Input: part model. Units: mm. Frame: model coordinates. Face numbers are marked on the shaded views. A direction names the side the tool comes from. Give positions to 0.01 mm unless a question says otherwise; leave off trailing zeros. Write each loop counter-clockwise with the first axis right and the second up, starting at its lowest first coordinate (ties: lowest second). Pieces come first, ordered by that corner, then holes. Notation, with made-up numbers: (45.25, 33.25) - (55.25, 33.25) arc R14 cw to (55.25, 46.25) - close; hole circle Ø8 at (60.5, -10.5). An arc over 180 degrees is marked (long way). Use a Markdown table: item, result. Add a question column.
1. Section query A-A, the plane x = -40. Return loops of the section in (y, z) (3 decimals), plus the area to 3 significant figures.
2. Pin query (flat end, axial travel): pin 1 (1.8 mm diameter, centred on y = 25, z = -2.5, fed in from +X); pin 2 (7.5 mm diameter, centred on x = 20.5, y = -31, fed in from +Z); pin 3 (3 mm diameter, centred on x = 42, z = -3.5, fed in from +Y). Return the tip coordinate at first contact, or that it passes through.
3. Set-up query: the marked faces 1, 2 and 3. Return all of +Z, -Z, +X, -X, +Y, -Y with unobstructed straight access to the full face (end or side cutting, diameter ignored); none if empty.
4. Material intervals for probe 1 along Y at (x, z) = (21.2, -4.7); probe 2 along Y at (x, z) = (-21.2, -3.95); probe 3 along Z at (x, y) = (30, 24.5), sorted ascending.
5. Section query B-B, the plane y = 0. Return loops of the section in (x, z) (3 decimals).
6. Section query C-C, the plane x = 21.2. Return loops of the section in (y, z).
7. Section query D-D, the plane x = -21.2. Return loops of the section in (y, z), plus the area to 3 significant figures.
```python
from build123d import *

# Parameters (mm, degrees)
F0_W     = 70
F0_H     = 40
F0_W_2   = 60
F0_H_2   = 7.5
F0_R     = 2.05
F0_R_2   = 2.125
F1_DEPTH = 6
F2_DEPTH = 3
F3_SIZE  = 1.5
F5_DEPTH = 2.5


with BuildPart() as f1:
    # F0 (on Top) → F1 (new body)
    with BuildSketch(Plane.XY):
        Rectangle(F0_W, F0_H)
        Rectangle(F0_W_2, F0_H_2, mode=Mode.SUBTRACT)
        with BuildLine():
            ThreePointArc((35, 27), (32.6568542495, 32.6568542495), (27, 35))
            Line((27, 35), (-27, 35))
            ThreePointArc((-27, 35), (-32.6568542495, 32.6568542495), (-35, 27))
            Line((-35, 27), (-35, 20))
            Line((-35, 20), (35, 20))
            Line((35, 20), (35, 27))
        make_face()
        with Locations((-21.2, 29)):
            Circle(F0_R, mode=Mode.SUBTRACT)
        with Locations((21.2, 29)):
            Circle(F0_R, mode=Mode.SUBTRACT)
        with BuildLine():
            Line((35, -27), (35, -20))
            Line((35, -20), (-35, -20))
            Line((-35, -20), (-35, -27))
            ThreePointArc((-35, -27), (-32.6568542495, -32.6568542495), (-27, -35))
            Line((-27, -35), (27, -35))
            ThreePointArc((27, -35), (32.6568542495, -32.6568542495), (35, -27))
        make_face()
        with Locations((-21.2, -29)):
            Circle(F0_R, mode=Mode.SUBTRACT)
        with Locations((21.2, -29)):
            Circle(F0_R, mode=Mode.SUBTRACT)
        with BuildLine():
            Line((45, 20), (35, 20))
            Line((35, 20), (35, -20))
            Line((35, -20), (45, -20))
            ThreePointArc((45, -20), (48.5355339059, -18.5355339059), (50, -15))
            Line((50, -15), (50, 15))
            ThreePointArc((50, 15), (48.5355339059, 18.5355339059), (45, 20))
        make_face()
        with Locations((40, 0)):
            Circle(F0_R_2, mode=Mode.SUBTRACT)
        with BuildLine():
            Line((-35, -20), (-35, 20))
            Line((-35, 20), (-45, 20))
            ThreePointArc((-45, 20), (-48.5355339059, 18.5355339059), (-50, 15))
            Line((-50, 15), (-50, -15))
            ThreePointArc((-50, -15), (-48.5355339059, -18.5355339059), (-45, -20))
            Line((-45, -20), (-35, -20))
        make_face()
        with Locations((-40, 0)):
            Circle(F0_R_2, mode=Mode.SUBTRACT)
        Rectangle(F0_W_2, F0_H_2)
        with Locations((-21.2, -29)):
            Circle(F0_R)
    extrude(amount=-F1_DEPTH)

    # F0 (on Top) → F2 (join)
    with BuildSketch(Plane.XY):
        Rectangle(F0_W_2, F0_H_2)
    extrude(amount=F2_DEPTH)

    # F3
    f3_edges = [f1.edges().sort_by_distance(p)[0] for p in [
        (-42.125, 0, -6),
        (37.875, 0, -6),
    ]]
    chamfer(f3_edges, length=F3_SIZE)

    # F4 (on Top) → F5 (cut)
    with BuildSketch(Plane.XY):
        Polygon((19.1289578016, -32.5574766695), (23.1704096859, -32.5574766695), (25.191135628, -29.0574766695), (23.1704096859, -25.5574766695), (19.1289578016, -25.5574766695), (17.1082318594, -29.0574766695), align=None)
        Polygon((-17.1082318594, -29.0574766695), (-19.1289578016, -25.5574766695), (-23.1704096859, -25.5574766695), (-25.191135628, -29.0574766695), (-23.1704096859, -32.5574766695), (-19.1289578016, -32.5574766695), align=None)
        Polygon((-23.1704096859, 25.5574766695), (-19.1289578016, 25.5574766695), (-17.1082318594, 29.0574766695), (-19.1289578016, 32.5574766695), (-23.1704096859, 32.5574766695), (-25.191135628, 29.0574766695), align=None)
        Polygon((19.1289578016, 32.5574766695), (17.1082318594, 29.0574766695), (19.1289578016, 25.5574766695), (23.1704096859, 25.5574766695), (25.191135628, 29.0574766695), (23.1704096859, 32.5574766695), align=None)
    extrude(amount=-F5_DEPTH, mode=Mode.SUBTRACT)


solid = f1.part
```
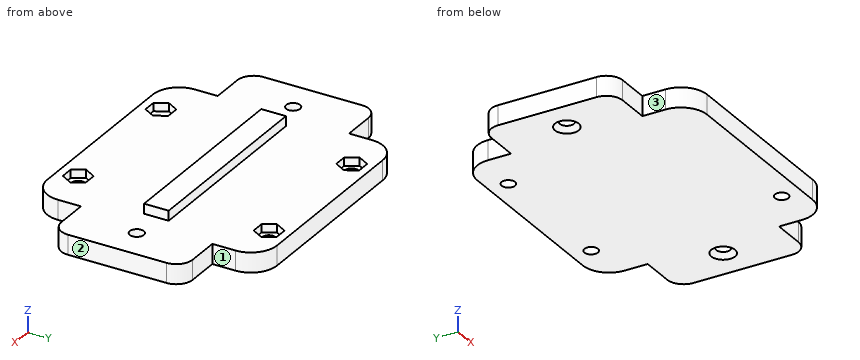
Result sheet:
| question | item | result |
|---|---|---|
| 1 | outline | (-20, -6) - (-3.625, -6) - (-2.125, -4.5) - (-2.125, 0) - (-20, 0) - close; (2.125, -4.5) - (3.625, -6) - (20, -6) - (20, 0) - (2.125, 0) - close |
| 1 | area | 212 mm² |
| 2 | pin 1 | stops at x = 35 |
| 2 | pin 2 | stops at z = 0 |
| 2 | pin 3 | stops at y = 20 |
| 3 | face 1 | +Z, -Z, +X, +Y |
| 3 | face 2 | +Z, -Z, +X, +Y, -Y |
| 3 | face 3 | +Z, -Z, -X, -Y |
| 4 | probe 1 | y = -35 to -31.05, -26.95 to 26.95, 31.05 to 35 |
| 4 | probe 2 | y = -35 to 26.95, 31.05 to 35 |
| 4 | probe 3 | z = -6 to 0 |
| 5 | outline | (-50, -6) - (-43.625, -6) - (-42.125, -4.5) - (-42.125, 0) - (-50, 0) - close; (-37.875, -4.5) - (-36.375, -6) - (36.375, -6) - (37.875, -4.5) - (37.875, 0) - (30, 0) - (30, 3) - (-30, 3) - (-30, 0) - (-37.875, 0) - close; (42.125, -4.5) - (43.625, -6) - (50, -6) - (50, 0) - (42.125, 0) - close |
| 6 | outline | (-35, -6) - (-31.05, -6) - (-31.05, -2.5) - (-32.56, -2.5) - (-32.56, 0) - (-35, 0) - close; (-26.95, -6) - (26.95, -6) - (26.95, -2.5) - (25.56, -2.5) - (25.56, 0) - (3.75, 0) - (3.75, 3) - (-3.75, 3) - (-3.75, 0) - (-25.56, 0) - (-25.56, -2.5) - (-26.95, -2.5) - close; (31.05, -6) - (35, -6) - (35, 0) - (32.56, 0) - (32.56, -2.5) - (31.05, -2.5) - close |
| 7 | outline | (-35, -6) - (26.95, -6) - (26.95, -2.5) - (25.56, -2.5) - (25.56, 0) - (3.75, 0) - (3.75, 3) - (-3.75, 3) - (-3.75, 0) - (-25.56, 0) - (-25.56, -2.5) - (-32.56, -2.5) - (-32.56, 0) - (-35, 0) - close; (31.05, -6) - (35, -6) - (35, 0) - (32.56, 0) - (32.56, -2.5) - (31.05, -2.5) - close |
| 7 | area | 393 mm² |
